Verification items for this drawing (mm, ordinates from the low corner). A direction names the side the tool comes from. Give positions to 0.01 mm unless a question says otherwise; leave off trailing zeros. Loops run counter-clockwise (first coordinate to the right, second up) from the corner with the lowest first, then second, coordinate; pieces in that order, holes last. Notation, with made-up numbers: M -14.75,63 L 43.25,63 A31 ccw 43.25,87 Z; hole C 53,75.25 d1. An arc over 180 degrees is marked long. Answer in a Markdown table with one row per item.
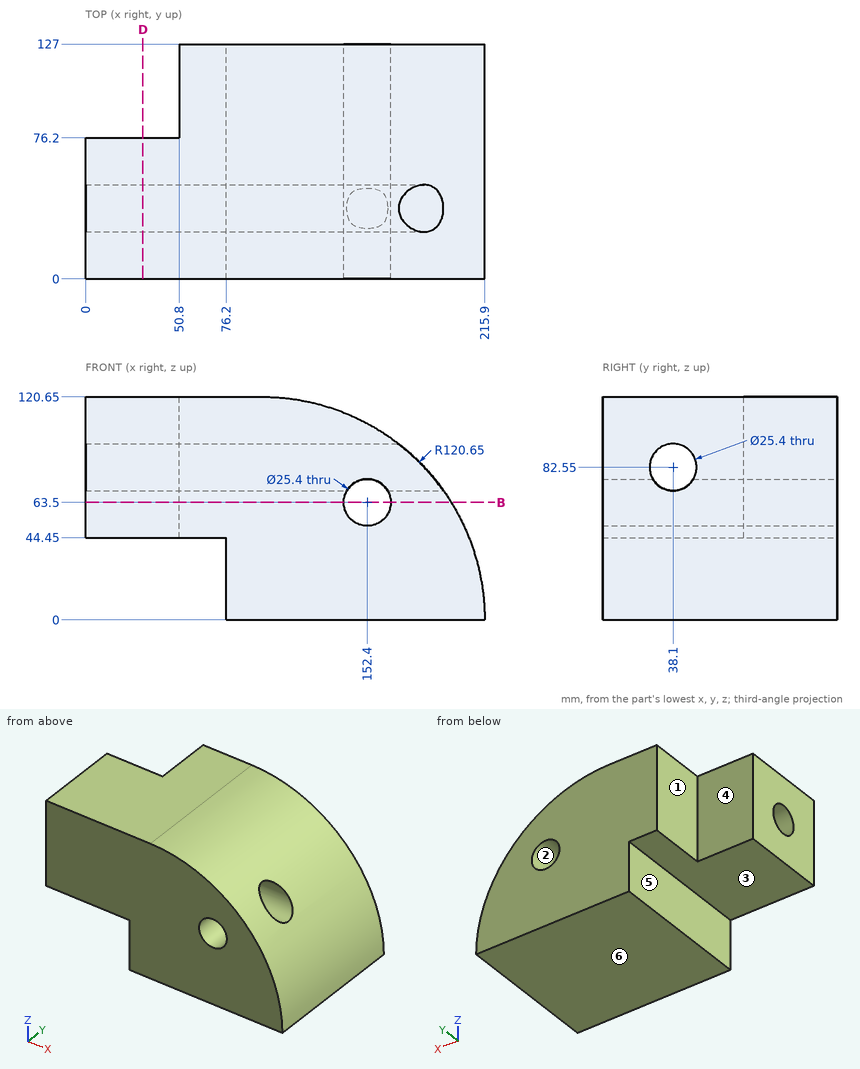
Item 1: Release check for a two-part mould opening along Z. For the marked faces 1, 2 and 3 record: released by +Z, released by -Z, zero draft, split by the parting line, or undercut.
Reported:
| item | result |
|---|---|
| face 1 | zero draft |
| face 2 | undercut |
| face 3 | released by -Z |
Item 2: Scan lines: L1, parallel to Z at x = 20, y = 21; L2, parallel to X at y = 52, z = 63; L3, parallel to Y at x = 32, z = 57. Record each from-to range of solid material in increasing order. Write a range as [from, to].
Reported:
| item | result |
|---|---|
| L1 | z = [44.45, 120.65] |
| L2 | x = [0, 139.71], [165.09, 198.15] |
| L3 | y = [0, 76.2] |
Item 3: Tool access check on the marked faces 4, 5 and 6. Record the directions out of +Z, -Z, +X, -X, +Y, -Y that give a thin tool (end or side, any length) a straight path to the whole face; none if there is none.
Reported:
| item | result |
|---|---|
| face 4 | +Z, -Z, -X, +Y |
| face 5 | -Z, -X, +Y, -Y |
| face 6 | -Z, +X, -X, +Y, -Y |
Item 4: Go/stop test with flat-tipped pins: pin 1 (1.5 mm diameter, centred on y = 33.5, z = 28, fed in from -X); pin 2 (12 mm diameter, centred on x = 125.5, y = 74, fed in from +Z); pin 3 (4 mm diameter, centred on y = 98.5, z = 54.5, fed in from -X). Record where each tip stops, or that it passes through.
Reported:
| item | result |
|---|---|
| pin 1 | stops at x = 76.2 |
| pin 2 | stops at z = 118.19 |
| pin 3 | stops at x = 50.8 |
Item 5: Sectioned sample at D-D (x = 31). Record the cut outline in (y, z), and give its area (3 significant figures).
Reported:
| item | result |
|---|---|
| outline | M 0,44.45 L 76.2,44.45 L 76.2,120.65 L 0,120.65 Z; hole C 38.1,82.55 d25.4 |
| area | 5,300 mm^2 |
Item 6: Sectioned sample at B-B (z = 63.5). Record the cut outline in (x, y), and give its area (3 significant figures).
Reported:
| item | result |
|---|---|
| outline | M 0,0 L 139.7,0 L 139.7,127 L 50.8,127 L 50.8,76.2 L 0,76.2 Z; M 165.1,0 L 197.84,0 L 197.84,127 L 165.1,127 Z |
| area | 19,300 mm^2 |
